from build123d import *

# Parameters (mm, degrees)
F0_R     = 3
F1_DEPTH = 37
F2_W     = 3
F2_H     = 19
F2_H_2   = 6
F3_DEPTH = 12.5
F4_SIZE  = 0.5
F5_R     = 0.5


with BuildPart() as f1:
    # F0 (on Top) → F1 (new body)
    with BuildSketch(Plane.XY):
        Circle(F0_R)
    extrude(amount=F1_DEPTH)

    # F2 (on Front) → F3 (cut, symmetric)
    with BuildSketch(Plane.XZ):
        with Locations((-1.5, 24.5)):
            Rectangle(F2_W, F2_H)
        with Locations((-1.5, 5.5)):
            Rectangle(F2_W, F2_H_2)
    extrude(amount=F3_DEPTH, both=True, mode=Mode.SUBTRACT)

    # F4
    f4_edges = [f1.edges().sort_by_distance(p)[0] for p in [
        (-3, 0, 37),
        (-3, 0, 0),
    ]]
    chamfer(f4_edges, length=F4_SIZE)

    # F5
    f5_edges = [f1.edges().sort_by_distance(p)[0] for p in [
        (0, 0, 8.5),
        (0, 0, 2.5),
        (0, 0, 15),
        (0, 0, 34),
    ]]
    fillet(f5_edges, radius=F5_R)


solid = f1.part
Verification items for the finished model (mm, model axes). A direction names the side the tool comes from. Coordinates: 2 decimals unless noted, no trailing zeros. Write each loop counter-clockwise with the first axis right and the second up, starting at its lowest first coordinate (ties: lowest second). Pieces come first, ordered by that corner, then holes. Notation, with made-up numbers: M 27,40 L 45,40 A20 ccw 45,71 Z; hole C -40,-36.5 d1. An arc over 180 degrees is marked long. Use CSV: the item, a comma, the result in double quotes.
Q1. Section check C-C, the plane z = 10. Enter the section's corners in (x, y), and give its area (3 significant figures).
Computed values:
outline,"C 0,0 d6"
area,"28.3 mm²"
Q2. Section check B-B, the plane z = 27. Enter the section's corners in (x, y).
Computed values:
outline,"M 0,-3 A3 ccw 0,3 Z"
Q3. Thickness scan on line 1 along Z through (x, y) = (-0.75, -1.5); line 2 along Z through (x, y) = (-2, -2); line 3 along X through (y, z) = (0, 3). Record the ranges inside material, lowest first. Write a range as [from, to].
Computed values:
line 1,"[0, 2.5], [8.5, 15], [34, 37]"
line 2,"[0.33, 2.5], [8.5, 15], [34, 36.67]"
line 3,"[0, 3]"
Q4. Set-up check for faces 1 (the cylindrical face through (2.77, -1.15, 18.25)), 2 (the flat face through (-1, 0, 2.5)): record each of +Z, -Z, +X, -X, +Y, -Y from which the full face is reachable in a straight line by a thin tool's end or side.
Computed values:
face 1,"+Z, -Z"
face 2,"-X, +Y, -Y"
Q5. Go/stop test with flat-tipped pins: P1, Ø1, axis at x = 2, z = 20, coming from the -Y side; P2, Ø1, axis at x = 1, z = 25.5, coming from the +Y side. Record where each tip stops, or that it passes through.
Computed values:
P1,"y = -2.6"
P2,"y = 2.96"
Q6. Section check A-A, the plane y = 0. Enter the section's corners in (x, z), and give its area (3 significant figures).
Computed values:
outline,"M -3,0.5 L -2.5,0 L 2.5,0 L 3,0.5 L 3,36.5 L 2.5,37 L -2.5,37 L -3,36.5 L -3,34 L -0.5,34 A0.5 cw 0,33.5 L 0,15.5 A0.5 cw -0.5,15 L -3,15 L -3,8.5 L -0.5,8.5 A0.5 cw 0,8 L 0,3 A0.5 cw -0.5,2.5 L -3,2.5 Z"
area,"147 mm²"
Q7. Mould release check, pull along Z, two halves, no side actions. Record for faces 3 (the flat face through (0, 0, 0)), 4 (the flat face through (0, 0, 24)), 5 (the flat face through (0, 0, 37)), 6 (the flat face through (-1, 0, 8.5)): pulls with the +Z half, pulls with the -Z half, needs draft (parallel to the pull), parting line crosses it, or undercut.
Computed values:
face 3,"pulls with the -Z half"
face 4,"undercut"
face 5,"pulls with the +Z half"
face 6,"undercut"
